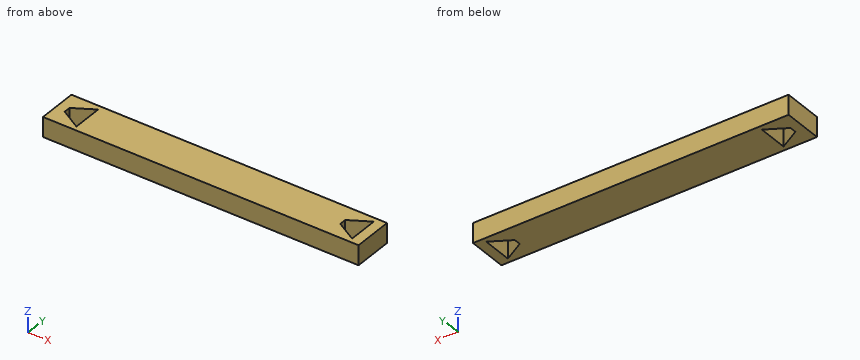
from build123d import *

# Parameters (mm, degrees)
SKETCH_W     = 160
SKETCH_H     = 20
PAD_DEPTH    = 10
POCKET_DEPTH = 10


with BuildPart() as part:
    # Sketch → Pad (new body)
    with BuildSketch(Plane.XY):
        with Locations((7.304336, 4.746988)):
            Rectangle(SKETCH_W, SKETCH_H)
    extrude(amount=PAD_DEPTH)

    # Sketch001 (on Face6 of Pad) → Pocket (cut)
    with BuildSketch(Plane.XY.offset(10)):
        Polygon((-67.695664, 3.039828), (-67.695664, 6.454148), (-57.445664, 12.371988), (-57.445664, -2.878012), align=None)
        Polygon((72.054336, 3.039828), (72.054336, 6.454148), (82.304336, 12.371988), (82.304336, -2.878012), align=None)
    extrude(amount=-POCKET_DEPTH, mode=Mode.SUBTRACT)


solid = part.part
The listing builds one solid part. Answer for the finished solid, in the listing's coordinates (mm). Round coordinates to 2 decimals unless told otherwise and drop trailing zeros. Write each loop counter-clockwise with the first axis right and the second up, starting at its lowest first coordinate (ties: lowest second). Pieces come first, ordered by that corner, then holes. Notation, with made-up numbers: (12, 64) - (41, 64) arc R22 ccw to (41, 70) - close; hole circle Ø7 at (3, 31.25). An arc over 180 degrees is marked (long way). Use a Markdown table: item, result. Add a question column.
1. The part is cut by section A-A (z = 2.5). Write down the section's boundary in (x, y).
2. The part is cut by section B-B (y = 4.75). Write down the section's boundary in (x, z), and give its area (4 significant figures).
3. Consider line 1 (X direction, y = 6, z = 0.5); line 2 (X direction, y = 12.25, z = 7.75); line 3 (Y direction, x = 80.5, z = 1.25). Determine where each line is inside the solid, lowest interval first.
Reported:
| question | item | result |
|---|---|---|
| 1 | outline | (-72.7, -5.25) - (87.3, -5.25) - (87.3, 14.75) - (-72.7, 14.75) - close; hole (-67.7, 3.04) - (-57.45, -2.88) - (-57.45, 12.37) - (-67.7, 6.45) - close; hole (72.05, 3.04) - (82.3, -2.88) - (82.3, 12.37) - (72.05, 6.45) - close |
| 2 | outline | (-72.7, 0) - (-67.7, 0) - (-67.7, 10) - (-72.7, 10) - close; (-57.45, 0) - (72.05, 0) - (72.05, 10) - (-57.45, 10) - close; (82.3, 0) - (87.3, 0) - (87.3, 10) - (82.3, 10) - close |
| 2 | area | 1,395 mm^2 |
| 3 | line 1 | -72.7 to -67.7, -57.45 to 72.05, 82.3 to 87.3 |
| 3 | line 2 | -72.7 to -57.66, -57.45 to 82.09, 82.3 to 87.3 |
| 3 | line 3 | -5.25 to -1.84, 11.33 to 14.75 |
